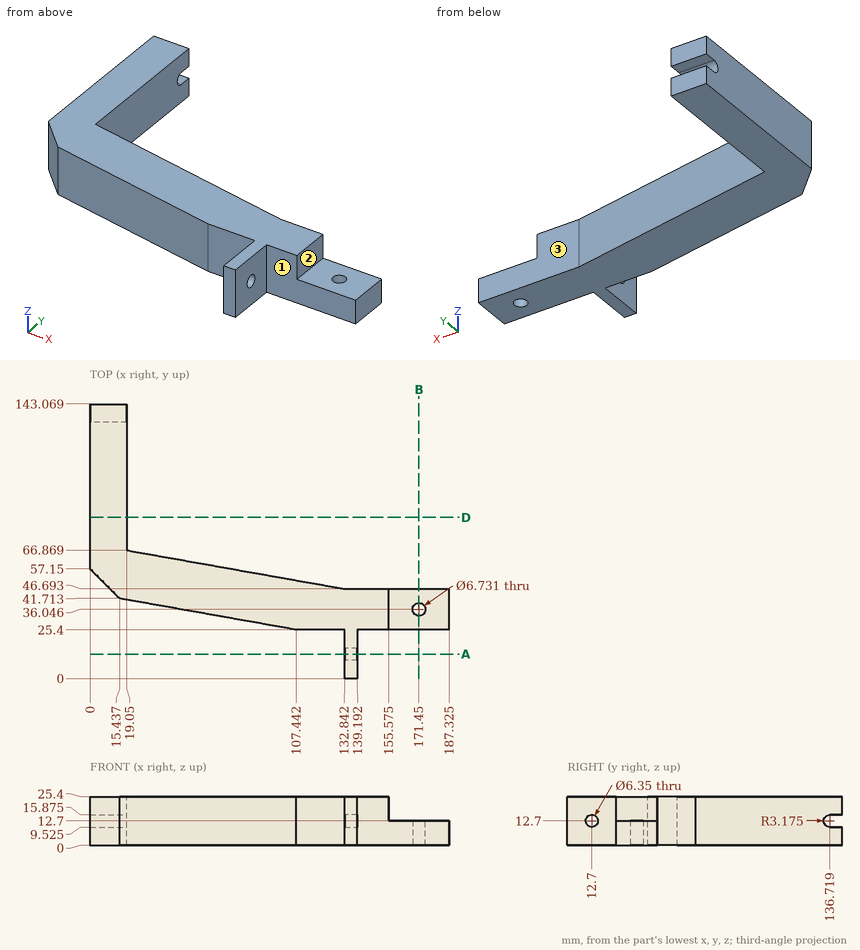
For this review, use the dimensioned drawing (mm, ordinates from the lowest corner) and the shaded views. A direction names the side the tool comes from. Coordinates: 2 decimals unless noted, no trailing zeros. Order: outer loops, then holes, each group sorted by start corner. A loop starts at its lowest first (then second) coordinate and runs counter-clockwise, first axis right, second up. Notation, with made-up numbers: (42.5, 27) - (63.5, 27) arc R21 ccw to (63.5, 36) - close; hole circle Ø8 at (-23.75, 36.5). An arc over 180 degrees is marked (long way). Answer as a JSON object with one key per item and string values. Group by question number.
1. For the marked faces 1, 2 and 3, list the 3-axis set-ups (+Z, -Z, +X, -X, +Y, -Y) from which the entire face can be reached by the end or side of a thin tool; tool diameter is ignored.
2. Clearance check with flat-ended pins moving along their axes: P1, Ø1.5, axis at y = 41, z = 9.5, coming from the -X side; P2, Ø4, axis at y = 12.7, z = 12.7, coming from the +X side; P3, Ø1.5, axis at y = 82.5, z = 6.5, coming from the +X side; P4, Ø12.5, axis at y = 16, z = 8, coming from the +X side. State where each tip first meets the part, or that it passes through.
3. We need section A-A on y = 12.7. State the section outline as (x, z) points (1 decimal).
4. We need section B-B on x = 171.45. State the section outline as (y, z) points, then the cut area to 3 significant figures.
5. We need section D-D on y = 84. State the section outline as (x, z) points.
6. For probe 1 along Y at (x, z) = (136, 12.7) (1 decimal); probe 2 along Z at (x, y) = (136.25, 12.7) (1 decimal); probe 3 along Y at (x, z) = (171.45, 9.75), list the stretches that pass through material, from the lowest coordinate up.
Final values:
{
 "1": {"face 1": "+Z, -Z, +X, -Y", "face 2": "+Z, +X, +Y, -Y", "face 3": "+Z, -Z, +X, +Y"},
 "2": {"P1": "x = 15.4", "P2": "through", "P3": "x = 19.05", "P4": "x = 139.19"},
 "3": {"outline": "(132.8, 0) - (139.2, 0) - (139.2, 9.5) - (132.8, 9.5) - close; (132.8, 15.9) - (139.2, 15.9) - (139.2, 25.4) - (132.8, 25.4) - close"},
 "4": {"outline": "(25.4, 0) - (32.68, 0) - (32.68, 12.7) - (25.4, 12.7) - close; (39.41, 0) - (46.69, 0) - (46.69, 12.7) - (39.41, 12.7) - close", "area": "185 mm²"},
 "5": {"outline": "(0, 0) - (19.05, 0) - (19.05, 25.4) - (0, 25.4) - close"},
 "6": {"probe 1": "0 to 9.5, 15.9 to 46.7", "probe 2": "0 to 9.5, 15.9 to 25.4", "probe 3": "25.4 to 32.68, 39.41 to 46.69"}
}
